Geometry: final body of the model. Coordinates: model frame, mm. A direction names the side the tool comes from. Coordinates: 2 decimals unless noted, no trailing zeros. Order: outer loops, then holes, each group sorted by start corner. A loop starts at its lowest first (then second) coordinate and runs counter-clockwise, first axis right, second up. Notation, with made-up numbers: (34.25, 50) -> (79.25, 50) arc R9 ccw to (79.25, 66) -> close; hole circle Ø3 at (24, 82.5). An arc over 180 degrees is marked (long way). Answer in a Markdown table with one row per item. Add a question column.
1) Contact query for flat-ended pins moving along their axis: P1, Ø2, axis at x = 9, y = 12.5, coming from the +Z side; P2, Ø1.5, axis at x = -7.5, z = -0.5, coming from the -Y side; P3, Ø4, axis at x = 2, z = -4, coming from the +Y side. Output: stop coordinate, or through.
2) Section query B-B on z = 0. Return the cut outline in (x, y), then the cut area to 3 significant figures.
3) Section query A-A on x = 0. Return the cut outline in (y, z), then the cut area to 3 significant figures.
4) Set-up query: faces 1 (the face through (-0.215, 24.636, -9.61)), 2 (the face through (5, 4, -3.15)), 3 (the face through (-0.04, 3.45, 3.95)), 4 (the face through (0, 7, 5)). Return all of +Z, -Z, +X, -X, +Y, -Y with unobstructed straight access to the full face (end or side cutting, diameter ignored); none if empty.
5) Ray query, line 1 (Y direction, x = 0, z = -8.05); line 2 (X direction, y = 16.75, z = 0). Return the intervals inside material, ascending. Write a range as from..to.
6) Section query C-C on x = -5.75. Return the cut outline in (y, z), then the cut area to 3 significant figures.
7) Pull-direction query (X, two-part tool) for faces 5 (the face through (11.923, 14.79, -3.755)), 6 (the face through (0.04, 3.45, -3.95)), 7 (the face through (5.4, 30, 5.4)); classes: +X half, -X half, draft (parallel to the pull), parting line (faces both ways), or undercut.
8) Section query D-D on y = 13. Return the cut outline in (x, z), then the cut area to 3 significant figures.
```python
from build123d import *

# Parameters (mm, degrees)
SKETCH1_R           = 12.5
BOSS_EXTRUDE1_DEPTH = 30
SKETCH2_R           = 7
CUT_EXTRUDE1_DEPTH  = 23
CUT_EXTRUDE3_DEPTH  = 7.6
SKETCH6_R           = 1
CUT_EXTRUDE4_DEPTH  = 7.6
FILLET2_R           = 1
SKETCH7_R           = 1.65
CUT_EXTRUDE5_DEPTH  = 19.5


with BuildPart() as part:
    # Sketch1 → Boss-Extrude1 (new body)
    with BuildSketch(Plane(origin=(0, 0, 0), x_dir=(1, 0, 0), z_dir=(0, 1, 0))):
        Circle(SKETCH1_R)
    extrude(amount=BOSS_EXTRUDE1_DEPTH)

    # Sketch2 → Cut-Extrude1 (cut)
    with BuildSketch(Plane(origin=(0, 30, 0), x_dir=(1, 0, 0), z_dir=(0, 1, 0))):
        Circle(SKETCH2_R)
    extrude(amount=-CUT_EXTRUDE1_DEPTH, mode=Mode.SUBTRACT)

    # Sketch5 → Cut-Extrude3 (cut)
    with BuildSketch(Plane(origin=(0, 0, 0), x_dir=(-1, 0, 0), z_dir=(0, -1, 0))):
        with BuildLine():
            Line((2.383275058, 3.15), (8.803408431, 3.15))
            ThreePointArc((8.803408431, 3.15), (9.35, 0), (8.803408431, -3.15))
            Line((8.803408431, -3.15), (2.383275058, -3.15))
            ThreePointArc((2.383275058, -3.15), (0, -3.95), (-2.383275058, -3.15))
            Line((-2.383275058, -3.15), (-8.803408431, -3.15))
            ThreePointArc((-8.803408431, -3.15), (-9.35, 0), (-8.803408431, 3.15))
            Line((-8.803408431, 3.15), (-2.383275058, 3.15))
            ThreePointArc((-2.383275058, 3.15), (0, 3.95), (2.383275058, 3.15))
        make_face()
    extrude(amount=-CUT_EXTRUDE3_DEPTH, mode=Mode.SUBTRACT)

    # Sketch6 → Cut-Extrude4 (cut)
    with BuildSketch(Plane.XZ):
        with Locations((-8.167012328, 2.513603897)):
            Circle(SKETCH6_R)
        with Locations((8.167012328, 2.513603897)):
            Circle(SKETCH6_R)
        with Locations((8.167012328, -2.513603897)):
            Circle(SKETCH6_R)
        with Locations((-8.167012328, -2.513603897)):
            Circle(SKETCH6_R)
    extrude(amount=-CUT_EXTRUDE4_DEPTH, mode=Mode.SUBTRACT)

    # Fillet2
    fillet2_edges = [part.edges().sort_by_distance(p)[0] for p in [
        (-9.099116447, 3.8, 2.151413462),
        (-7.395649897, 3.8, 3.15),
        (9.099116447, 3.8, -2.151413462),
        (9.099116447, 3.8, 2.151413462),
        (-9.099116447, 3.8, -2.151413462),
        (7.395649897, 3.8, 3.15),
        (7.395649897, 3.8, -3.15),
        (-7.395649897, 3.8, -3.15),
    ]]
    fillet(fillet2_edges, radius=FILLET2_R)

    # Sketch7 → Cut-Extrude5 (cut)
    with BuildSketch(Plane.XY):
        with Locations((0, 23)):
            Circle(SKETCH7_R)
    extrude(amount=-CUT_EXTRUDE5_DEPTH, mode=Mode.SUBTRACT)


solid = part.part
```
Result:
| question | item | result |
|---|---|---|
| 1 | P1 | z = 9.6 |
| 1 | P2 | y = 7.6 |
| 1 | P3 | y = 7 |
| 2 | outline | (-12.5, 0) -> (-9.35, 0) -> (-9.35, 7.6) -> (-7, 7.6) -> (-7, 30) -> (-12.5, 30) -> close; (7, 7.6) -> (9.35, 7.6) -> (9.35, 0) -> (12.5, 0) -> (12.5, 30) -> (7, 30) -> close |
| 2 | area | 294 mm2 |
| 3 | outline | (0, -12.5) -> (21.35, -12.5) -> (21.35, -7) -> (7, -7) -> (7, -3.95) -> (0, -3.95) -> close; (0, 3.95) -> (7, 3.95) -> (7, 7) -> (30, 7) -> (30, 12.5) -> (0, 12.5) -> close; (24.65, -12.5) -> (30, -12.5) -> (30, -7) -> (24.65, -7) -> close |
| 3 | area | 355 mm2 |
| 4 | face 1 | -Z |
| 4 | face 2 | -Y |
| 4 | face 3 | +Y, -Y |
| 4 | face 4 | +Y |
| 5 | line 1 | 0..21.35, 24.65..30 |
| 5 | line 2 | -12.5..-7, 7..12.5 |
| 6 | outline | (0, -11.1) -> (30, -11.1) -> (30, -3.99) -> (7, -3.99) -> (7, -3.15) -> (0, -3.15) -> close; (0, 3.15) -> (7, 3.15) -> (7, 3.99) -> (30, 3.99) -> (30, 11.1) -> (0, 11.1) -> close |
| 6 | area | 438 mm2 |
| 7 | face 5 | parting line |
| 7 | face 6 | undercut |
| 7 | face 7 | draft |
| 8 | outline | circle Ø25 at (0, 0); hole circle Ø14 at (0, 0) |
| 8 | area | 337 mm2 |
